Can you work these out from the model? Positions are in its coordinate system, mm. A direction names the side the tool comes from. Round coordinates to 2 decimals unless told otherwise and drop trailing zeros. Loops run counter-clockwise (first coordinate to the right, second up) from the corner with the lowest first, then second, coordinate; pieces in that order, holes last. Notation, with made-up numbers: (-15.5, -23.5) -> (11.5, -23.5) arc R9 ccw to (11.5, -14.5) -> close; hole circle Ø10 at (32, -9.5). An arc over 180 degrees is marked (long way). Use a Markdown table: item, result.
from build123d import *

# Parameters (mm, degrees)
SKETCH_W     = 99
SKETCH_H     = 81
PAD_DEPTH    = 25
THICKNESS_T  = 3
SKETCH004_R  = 1.6
POCKET_DEPTH = 40.001


with BuildPart() as part:
    # Sketch → Pad (new body)
    with BuildSketch(Plane.XY):
        with Locations((20, -91.5)):
            Rectangle(SKETCH_W, SKETCH_H)
    extrude(amount=PAD_DEPTH)

    # Thickness
    thickness_openings = [part.faces().sort_by_distance(p)[0] for p in [
        (20, -91.5, 25),
    ]]
    offset(amount=THICKNESS_T, openings=thickness_openings)

    # Sketch004 (on Part__Feature) → Pocket (cut, through all)
    with BuildSketch(Plane(origin=(-200, 0, 37), x_dir=(1, 0, 0), z_dir=(0, 0, 1))):
        with Locations((180, -63)):
            Circle(SKETCH004_R)
        with Locations((254, -124)):
            Circle(SKETCH004_R)
    extrude(amount=-POCKET_DEPTH, mode=Mode.SUBTRACT)


solid = part.part
1. I need wall thicknesses on line 1 (Y direction, x = -11.5, z = 16.25); line 2 (X direction, y = -88.5, z = 12.75); line 3 (Z direction, x = 33, y = -117). Which ranges of each line are inside material? Lowest first, please.
Answer sheet:
| item | result |
|---|---|
| line 1 | y = -135 to -132, -51 to -48 |
| line 2 | x = -32.5 to -29.5, 69.5 to 72.5 |
| line 3 | z = -3 to 0 |
2. I want a section at D-D (z = 5). Please give me the cut outline in (x, y).
Answer sheet:
| item | result |
|---|---|
| outline | (-32.5, -132) arc R3 ccw to (-29.5, -135) -> (69.5, -135) arc R3 ccw to (72.5, -132) -> (72.5, -51) arc R3 ccw to (69.5, -48) -> (-29.5, -48) arc R3 ccw to (-32.5, -51) -> close; hole (-29.5, -132) -> (69.5, -132) -> (69.5, -51) -> (-29.5, -51) -> close |
3. I want a section at B-B (y = -124). Please give me the cut outline in (x, z), plus the area to 3 significant figures.
Answer sheet:
| item | result |
|---|---|
| outline | (-32.5, 0) arc R3 ccw to (-29.5, -3) -> (52.4, -3) -> (52.4, 0) -> (-29.5, 0) -> (-29.5, 25) -> (-32.5, 25) -> close; (55.6, -3) -> (69.5, -3) arc R3 ccw to (72.5, 0) -> (72.5, 25) -> (69.5, 25) -> (69.5, 0) -> (55.6, 0) -> close |
| area | 452 mm² |
4. Which directions (+Z, -Z, +X, -X, +Y, -Y) give clear straight access to the entire face, cutting with the end or side of a thin tool? Please do faces 4 (the cylindrical face through (20.69, -48.86, -2.1)), 5 (the flat face through (69.5, -92, 12)).
Answer sheet:
| item | result |
|---|---|
| face 4 | -Z, +X, -X, +Y |
| face 5 | +Z |
5. Will this pin go through, and if not, where does the flat tip stop? pin 1 Ø1.9 at (x, y) = (-20, -63) entering from -Z.
Answer sheet:
| item | result |
|---|---|
| pin 1 | passes through |
6. If we mould it in two halves opening along Y, with no side actions, what happens to faces 1 (the cylindrical face through (20.69, -134.14, -2.1)), 2 (the flat face through (-32.5, -92, 12)), 3 (the cylindrical face through (-20.208, -61.414, -1.479))? For each: +Y half, -Y half, draft (parallel to the pull), parting line (faces both ways), or undercut.
Answer sheet:
| item | result |
|---|---|
| face 1 | -Y half |
| face 2 | draft |
| face 3 | undercut |
7. I want a section at C-C (y = -55). Please give me the cut outline in (x, z).
Answer sheet:
| item | result |
|---|---|
| outline | (-32.5, 0) arc R3 ccw to (-29.5, -3) -> (69.5, -3) arc R3 ccw to (72.5, 0) -> (72.5, 25) -> (69.5, 25) -> (69.5, 0) -> (-29.5, 0) -> (-29.5, 25) -> (-32.5, 25) -> close |
8. I want a section at A-A (x = -20). Please give me the cut outline in (y, z).
Answer sheet:
| item | result |
|---|---|
| outline | (-135, 0) arc R3 ccw to (-132, -3) -> (-64.6, -3) -> (-64.6, 0) -> (-132, 0) -> (-132, 25) -> (-135, 25) -> close; (-61.4, -3) -> (-51, -3) arc R3 ccw to (-48, 0) -> (-48, 25) -> (-51, 25) -> (-51, 0) -> (-61.4, 0) -> close |
